Check sheet for the drawn part. Datum: minimum x, y, z corner. Units: mm. A direction names the side the tool comes from. Round coordinates to 2 decimals unless told otherwise and drop trailing zeros. Loops run counter-clockwise (first coordinate to the right, second up) from the corner with the lowest first, then second, coordinate; pieces in that order, holes last.
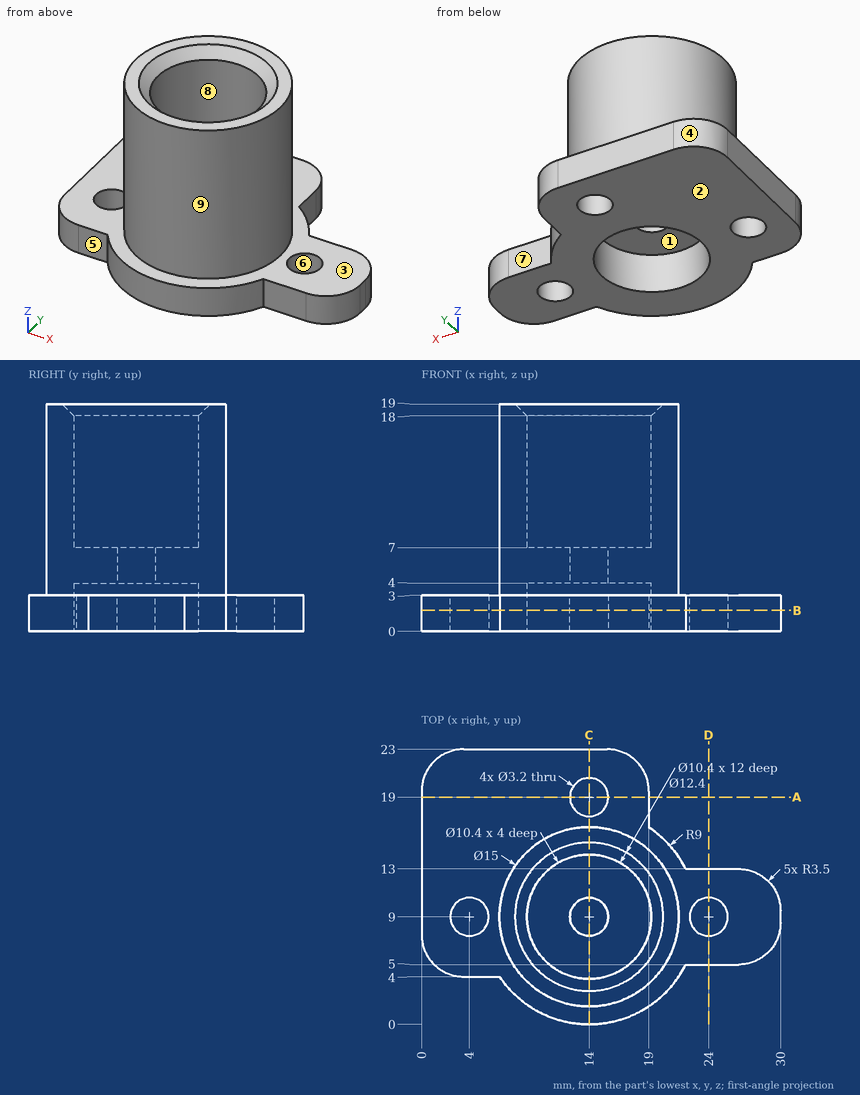
1) Access from +Z, -Z, +X, -X, +Y, -Y to the whole of each face (thin tool, end or side, straight path). Record for the marked faces 1, 2, 3, 4 and 5.
Report:
face 1: -Z
face 2: -Z, +X, -X, +Y, -Y
face 3: +Z
face 4: +Z, -Z, -X, +Y
face 5: +Z, -Z, -X, -Y
2) Gauge pin test, flat ends, axial feed: pin 1 (2.5 mm diameter, centred on y = 17.5, z = 1.5, fed in from +X); pin 2 (3.5 mm diameter, centred on x = 4.5, z = 1.5, fed in from -Y); pin 3 (2 mm diameter, centred on x = 14, y = 10.5, fed in from -Z); pin 4 (1 mm diameter, centred on y = 18, z = 7, fed in from -X). Record the tip position at first contact, or that the pin passes through.
Report:
pin 1: stops at x = 19.33
pin 2: stops at y = 4
pin 3: stops at z = 4
pin 4: passes through
3) Sectioned sample at C-C, the plane x = 14. Record the cut outline in (y, z).
Report:
outline: (0, 0) - (3.8, 0) - (3.8, 4) - (7.4, 4) - (7.4, 7) - (3.8, 7) - (3.8, 18) - (2.8, 19) - (1.5, 19) - (1.5, 3) - (0, 3) - close; (10.6, 4) - (14.2, 4) - (14.2, 0) - (17.4, 0) - (17.4, 3) - (16.5, 3) - (16.5, 19) - (15.2, 19) - (14.2, 18) - (14.2, 7) - (10.6, 7) - close; (20.6, 0) - (23, 0) - (23, 3) - (20.6, 3) - close
4) Scan lines: line 1 along Y through (x, z) = (14, 2.45); line 2 along Y through (x, z) = (24, 1.75); line 3 along Z through (x, y) = (6.75, 13.5). Record each from-to range of solid material in increasing order.
Report:
line 1: y = 0 to 3.8, 14.2 to 17.4, 20.6 to 23
line 2: y = 5 to 7.4, 10.6 to 13
line 3: z = 0 to 3
5) Mould release check, pull along Y, two halves, no side actions. Record for the marked faces 6, 7, 8 and 9: +Y half, -Y half, draft (parallel to the pull), parting line (faces both ways), or undercut.
Report:
face 6: undercut
face 7: +Y half
face 8: undercut
face 9: parting line
6) Sectioned sample at B-B, the plane z = 1.75. Record the cut outline in (x, y).
Report:
outline: (0, 7.5) arc R3.5 ccw to (3.5, 4) - (6.52, 4) arc R9 ccw to (22.06, 5) - (26.5, 5) arc R3.5 ccw to (30, 8.5) - (30, 9.5) arc R3.5 ccw to (26.5, 13) - (22.06, 13) arc R9 ccw to (19, 16.48) - (19, 19.5) arc R3.5 ccw to (15.5, 23) - (3.5, 23) arc R3.5 ccw to (0, 19.5) - close; hole circle Ø3.2 at (4, 9); hole circle Ø10.4 at (14, 9); hole circle Ø3.2 at (14, 19); hole circle Ø3.2 at (24, 9)
7) Sectioned sample at A-A, the plane y = 19. Record the cut outline in (x, z), then the cut area to 3 significant figures.
Report:
outline: (0, 0) - (12.4, 0) - (12.4, 3) - (0, 3) - close; (15.6, 0) - (19, 0) - (19, 3) - (15.6, 3) - close
area: 47.4 mm2
8) Sectioned sample at D-D, the plane x = 24. Record the cut outline in (y, z).
Report:
outline: (5, 0) - (7.4, 0) - (7.4, 3) - (5, 3) - close; (10.6, 0) - (13, 0) - (13, 3) - (10.6, 3) - close
